from build123d import *

# Parameters (mm, degrees)
SKETCH003_R           = 35
SKETCH003_R_2         = 14
PAD002_DEPTH          = 3
SKETCH004_R           = 25
SKETCH004_R_2         = 23.5
POCKET001_DEPTH       = 1.7
POCKET002_DEPTH       = 201.081792
POLARPATTERN001_COUNT = 8
CHAMFER_SIZE          = 2


with BuildPart() as part:
    # Sketch003 → Pad002 (new body)
    with BuildSketch(Plane.XY):
        Circle(SKETCH003_R)
        Circle(SKETCH003_R_2, mode=Mode.SUBTRACT)
    extrude(amount=PAD002_DEPTH)

    # Sketch004 (on Face3 of Pad002) → Pocket001 (cut)
    with BuildSketch(Plane(origin=(0, 0, 0), x_dir=(1, 0, 0), z_dir=(0, 0, -1))):
        Circle(SKETCH004_R)
        Circle(SKETCH004_R_2, mode=Mode.SUBTRACT)
    extrude(amount=-POCKET001_DEPTH, mode=Mode.SUBTRACT)

    # Sketch005 (on Face2 of Pocket001) → Pocket002 (cut, through all)
    with BuildSketch(Plane(origin=(0, 0, 0), x_dir=(1, 0, 0), z_dir=(0, 0, -1))):
        with BuildLine():
            ThreePointArc((10.960155, 10.960155), (6.672922, 13.990072), (1.620191, 15.415089))
            ThreePointArc((1.72472, 16.409611), (1.175194, 15.964615), (1.620191, 15.415089))
            ThreePointArc((11.667262, 11.667262), (7.103433, 14.892657), (1.72472, 16.409611))
            ThreePointArc((10.960155, 10.960155), (11.667262, 10.960155), (11.667262, 11.667262))
        make_face()
        with BuildLine():
            ThreePointArc((13.788582, 13.788582), (8.394966, 17.600413), (2.038305, 19.393177))
            ThreePointArc((2.142833, 20.387699), (1.593308, 19.942702), (2.038305, 19.393177))
            ThreePointArc((14.495689, 14.495689), (8.825477, 18.502998), (2.142833, 20.387699))
            ThreePointArc((13.788582, 13.788582), (14.495689, 13.788582), (14.495689, 14.495689))
        make_face()
    pocket002 = extrude(amount=-POCKET002_DEPTH, mode=Mode.SUBTRACT)

    # PolarPattern001: Pocket002 ×8 about axis
    polarpattern001_axis = Axis((0, 0, 0), (0, 0, -1))
    for i in range(1, POLARPATTERN001_COUNT):
        add(pocket002.rotate(polarpattern001_axis, i * 360 / POLARPATTERN001_COUNT), mode=Mode.SUBTRACT)

    # Chamfer
    chamfer_edges = [part.edges().sort_by_distance(p)[0] for p in [
        (-35, 0, 3),
    ]]
    chamfer(chamfer_edges, length=CHAMFER_SIZE)


with BuildPart() as part_1:
    # Body001 placement: moved
    add(part.part.moved(Location((0, 0, 1.2))))


solid = part_1.part
Source: CAD feature listing. Evaluate the final solid. Frame: model axes, mm. A direction names the side the tool comes from. Coordinates: 2 decimals unless noted, no trailing zeros.
Item 1: Cut plane A-A (y = -8). Count the separate pieces of the cut face and the enclosed holes in it, plus the area to 3 significant figures.
Output values:
separate pieces: 6
enclosed holes: 0
area: 113 mm2
Item 2: First-contact query: P1, Ø25, axis at x = -2.5, y = 8, coming from the -Z side. Flat tip, straight axial feed; report the tip coordinate or a pass-through.
Output values:
P1: stops at z = 1.2
Item 3: Pull-direction query (X, two-part tool) for faces 4 (the face through (-24, 8, 1.2)), 5 (the face through (7.17, -14.86, 2.68)); classes: pulls with the +X half, pulls with the -X half, needs draft (parallel to the pull), parting line crosses it, or undercut.
Output values:
face 4: needs draft
face 5: undercut
Item 4: Material intervals for line 1 (Y direction, x = 17, z = 3.25); line 2 (X direction, y = -17, z = 3.8); line 3 (Y direction, x = 10.5, z = 4), sorted ascending.
Output values:
line 1: y = -29.39 to -11.46, -9.55 to 9.55, 11.46 to 29.39
line 2: x = -28.75 to -11.46, -9.55 to 9.55, 11.46 to 28.75
line 3: y = -31.5 to -17.61, -16.43 to -12.73, -11.4 to -9.26, 9.26 to 12.18, 12.69 to 16.43, 17.61 to 31.5
Item 5: Set-up query: faces 1 (the face through (-6.74, 13.96, 2.68)), 2 (the face through (23.846, -7.509, 2.038)), 3 (the face through (10.1, -10.1, 1.2)). Return all of +Z, -Z, +X, -X, +Y, -Y with unobstructed straight access to the full face (end or side cutting, diameter ignored); none if empty.
Output values:
face 1: +Z, -Z
face 2: -Z
face 3: -Z, +X, -X, +Y, -Y
